Here's how the part is built. I have some questions about the finished solid (model axes, mm). A direction names the side the tool comes from. Round coordinates to 2 decimals unless told otherwise and drop trailing zeros. Write each loop counter-clockwise with the first axis right and the second up, starting at its lowest first coordinate (ties: lowest second). Pieces come first, ordered by that corner, then holes. Notation, with made-up numbers: (24.25, -31.75) - (61.25, -31.75) arc R27 cw to (61.25, 7.25) - close; hole circle Ø7 at (-40, -3.75). An arc over 180 degrees is marked (long way). One line per question, with ' | ' between items. Start each with the question number.
(1) Will these pins go through, and if not, where does the flat tip stop? pin 1 (3 mm diameter, centred on y = -3, z = 11, fed in from +X) (3 decimals); pin 2 (6 mm diameter, centred on x = -20, y = 0.5, fed in from -Z); pin 3 (6 mm diameter, centred on x = -2, z = 12.5, fed in from +Y); pin 4 (7 mm diameter, centred on x = -35.92, y = -94.81, fed in from +Z).
(2) Imagine slicing it at B-B (y = 0). Write out the boundary of the cut face in (x, z), plus the area to 3 significant figures.
(3) If I drill on L1, parallel to Y at x = -19.5, z = 15.25; L2, parallel to Z at x = -41, y = -93.5; L3, parallel to Y at x = -35.5, z = 18.5, over which ranges is the centre line in solid material (lowest first)?
(4) Thinking about a two-plate mould opening in Y: for faces 5 (the cylindrical face through (-27.373, -65.165, 16.58)), 6 (the flat face through (-20, -135, 3.073)), which applies, pulls with the +Y half, pulls with the -Y half, needs draft (parallel to the pull), parting line crosses it, or undercut?
(5) Imagine slicing it at A-A (x = -19.5). Write out the boundary of the cut face in (y, z).
(6) For faces 1 (the cylindrical face through (-11.58, -64.23, 16.58)), 2 (the cylindrical face through (-47.994, -68.445, 14.608)), 3 (the cylindrical face through (-17.006, -1.034, 10.531)), 4 (the flat face through (-20, 0, 7.573)), which set-ups out of +Z, -Z, +X, -X, +Y, -Y let a thin tool reach every point of the face, with its end or its side?
from build123d import *

# Parameters (mm, degrees)
BOSS_EXTRUDE1_DEPTH      = 7
BOSS_EXTRUDE1_DEPTH_BACK = 5
SKETCH2_R                = 2.7
BOSS_EXTRUDE3_DEPTH      = 0.1
BOSS_EXTRUDE3_DEPTH_BACK = 6
CHAMFER1_SIZE            = 4
SKETCH5_R                = 2.7
BOSS_EXTRUDE4_DEPTH      = 6
CUT_EXTRUDE1_DEPTH       = 23
SKETCH7_R                = 2.7
CUT_EXTRUDE2_DEPTH       = 37
SKETCH8_R                = 6.25
BOSS_EXTRUDE5_DEPTH      = 2.5
SKETCH9_R                = 2.7
BOSS_EXTRUDE6_DEPTH      = 4.5


with BuildPart() as part:
    # Sketch2 → Boss-Extrude1 (new, two sides: drawn at the far end of the back side and taken through both)
    with BuildSketch(Plane.XY.offset(12.572663867).offset(-BOSS_EXTRUDE1_DEPTH_BACK)):
        with Locations((-19.5, 0)):
            Circle(SKETCH2_R)
    extrude(amount=BOSS_EXTRUDE1_DEPTH + BOSS_EXTRUDE1_DEPTH_BACK)

    # Sketch4 → Boss-Extrude3 (add, two sides: drawn at the far end of the back side and taken through both)
    with BuildSketch(Plane.XY.offset(19.572663867).offset(-BOSS_EXTRUDE3_DEPTH_BACK)):
        with BuildLine():
            ThreePointArc((16.476844134, -6.650636784), (-19.499999999, 36.586394787), (-55.476844134, -6.650636782))
            ThreePointArc((-55.476844134, -6.650636782), (-47.943109392, -69.328026103), (-48.367101444, -132.455140104))
            ThreePointArc((-48.367101444, -132.455140104), (-19.500000007, -163.413605213), (9.36710143, -132.455140104))
            ThreePointArc((9.36710143, -132.455140104), (8.943109385, -69.328026104), (16.476844134, -6.650636784))
        make_face()
    extrude(amount=BOSS_EXTRUDE3_DEPTH + BOSS_EXTRUDE3_DEPTH_BACK)

    # Chamfer1
    chamfer1_edges = [part.edges().sort_by_distance(p)[0] for p in [
        (-47.943109392, -69.328026103, 19.672663867),
        (-19.500000007, -163.413605213, 19.672663867),
        (8.943109385, -69.328026104, 19.672663867),
        (-19.499999999, 36.586394787, 19.672663867),
    ]]
    chamfer(chamfer1_edges, length=CHAMFER1_SIZE)

    # Sketch5 → Boss-Extrude4 (add)
    with BuildSketch(Plane(origin=(0, 0, 13.572663867), x_dir=(-1, 0, 0), z_dir=(0, 0, -1))):
        with Locations(Location((19.500000007, -134.475863937, 0), (0, 0, 180))):
            Circle(SKETCH5_R)
    extrude(amount=BOSS_EXTRUDE4_DEPTH)

    # Sketch6 → Cut-Extrude1 (cut)
    with BuildSketch(Plane(origin=(0, 0, 13.572663867), x_dir=(-1, 0, 0), z_dir=(0, 0, -1))):
        with BuildLine():
            ThreePointArc((30.487725375, -31.464034345), (19.500000001, -18.885340351), (8.512274628, -31.464034345))
            ThreePointArc((8.512274628, -31.464034345), (11.603309463, -64.698470815), (11.890013879, -98.075110316))
            ThreePointArc((11.890013879, -98.075110316), (19.500000005, -105.944284009), (27.109986131, -98.075110316))
            ThreePointArc((27.109986131, -98.075110316), (27.396690544, -64.698470815), (30.487725375, -31.464034345))
        make_face()
    extrude(amount=-CUT_EXTRUDE1_DEPTH, mode=Mode.SUBTRACT)

    # Sketch7 → Cut-Extrude2 (cut)
    with BuildSketch(Plane(origin=(0, 0, 13.572663867), x_dir=(-1, 0, 0), z_dir=(0, 0, -1))):
        with Locations((39.934899894, -33.677713254)):
            Circle(SKETCH7_R)
        with Locations((35.920760732, -94.813426318)):
            Circle(SKETCH7_R)
        with Locations((-0.934899891, -33.677713254)):
            Circle(SKETCH7_R)
        with Locations((3.079239271, -94.813426318)):
            Circle(SKETCH7_R)
    extrude(amount=-CUT_EXTRUDE2_DEPTH, mode=Mode.SUBTRACT)

    # Sketch8 → Boss-Extrude5 (add)
    with BuildSketch(Plane(origin=(0, 0, 13.572663867), x_dir=(-1, 0, 0), z_dir=(0, 0, -1))):
        with Locations(Location((19.500000007, -134.475863937, 0), (0, 0, 180))):
            Circle(SKETCH8_R)
    extrude(amount=BOSS_EXTRUDE5_DEPTH)

    # Sketch9 → Boss-Extrude6 (add)
    with BuildSketch(Plane(origin=(0, 0, 7.572663867), x_dir=(-1, 0, 0), z_dir=(0, 0, -1))):
        with Locations(Location((19.500000007, -134.475863937, 0), (0, 0, 180))):
            Circle(SKETCH9_R)
    extrude(amount=BOSS_EXTRUDE6_DEPTH)


solid = part.part
Check sheet entries:
1) pin 1: x = -17.255 | pin 2: z = 7.57 | pin 3: y = 33.5 | pin 4: z = 19.67
2) outline: (-56.09, 13.57) - (-22.2, 13.57) - (-22.2, 7.57) - (-16.8, 7.57) - (-16.8, 13.57) - (17.09, 13.57) - (17.09, 15.67) - (13.09, 19.67) - (-52.09, 19.67) - (-56.09, 15.67) - close | area: 463 mm^2
3) L1: -163.41 to -105.94, -18.89 to 36.59 | L2: 13.57 to 19.67 | L3: -155.11 to -97.48, -92.15 to 29.73
4) face 5: undercut | face 6: needs draft
5) outline: (-163.41, 13.57) - (-140.73, 13.57) - (-140.73, 11.07) - (-137.18, 11.07) - (-137.18, 3.07) - (-131.78, 3.07) - (-131.78, 11.07) - (-128.23, 11.07) - (-128.23, 13.57) - (-105.94, 13.57) - (-105.94, 19.67) - (-159.41, 19.67) - (-163.41, 15.67) - close; (-18.89, 13.57) - (-2.7, 13.57) - (-2.7, 7.57) - (2.7, 7.57) - (2.7, 13.57) - (36.59, 13.57) - (36.59, 15.67) - (32.59, 19.67) - (-18.89, 19.67) - close
6) face 1: +Z, -Z | face 2: +Z, -Z, -X | face 3: -Z | face 4: -Z, +X, -X, +Y
